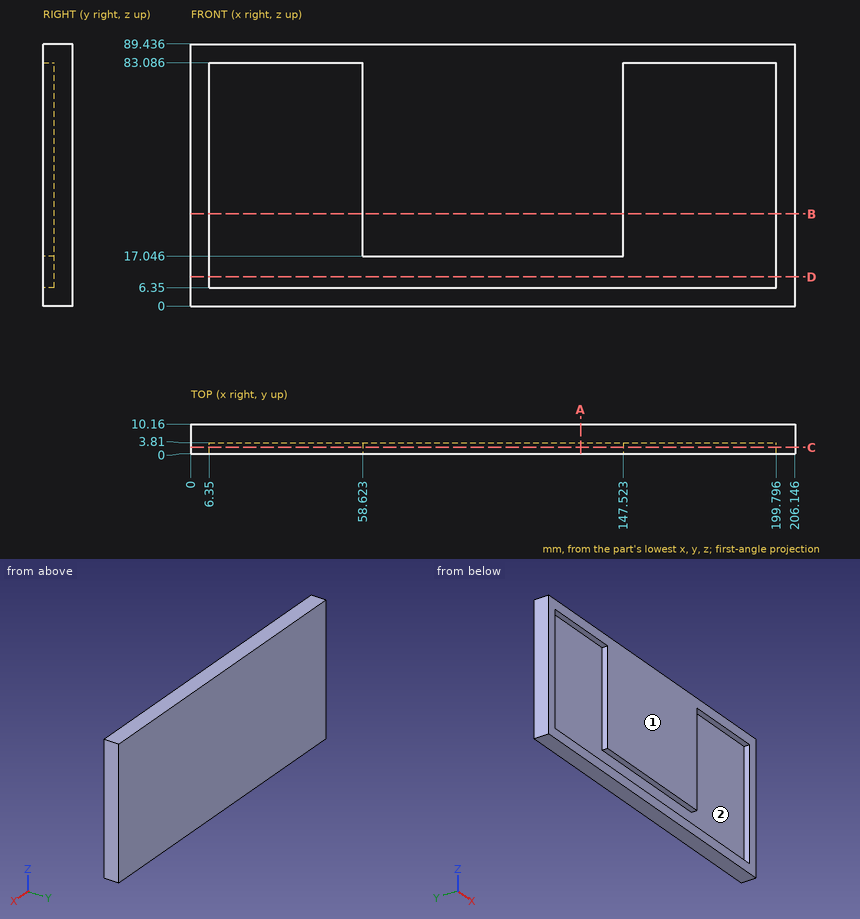
Part print with two shaded views. Sizes in mm from the minimum x, y, z corner. Give positions to 0.01 mm unless a question says otherwise; leave off trailing zeros. Order: outer loops, then holes, each group sorted by start corner. A loop starts at its lowest first (then second) coordinate and runs counter-clockwise, first axis right, second up. Notation, with made-up numbers: M 23.25,-18.5 L 69.25,-18.5 A21 cw 69.25,15.5 Z; hole C -1,6.5 d7. An arc over 180 degrees is marked long. Put each result on its own line as item: value.
Item 1: Pull direction X, two halves, no side cores. Call the marked faces 1 and 2: +X half, -X half, draft (parallel to the pull), parting line (faces both ways), or undercut.
Results are:
face 1: draft
face 2: undercut
Item 2: Drop flat-ended pins along their axis: pin 1 Ø3 at (x, y) = (104.5, 4.5) entering from -Z; pin 2 Ø3 at (x, z) = (178.5, 52) entering from -Y. Give the stop position or say it passes through.
Results are:
pin 1: z = 0
pin 2: y = 3.81
Item 3: Cut at D-D on z = 10. Write the cut outline in (x, y), then the cut area to 3 significant figures.
Results are:
outline: M 0,0 L 6.35,0 L 6.35,3.81 L 199.8,3.81 L 199.8,0 L 206.15,0 L 206.15,10.16 L 0,10.16 Z
area: 1,360 mm2
Item 4: Cut at B-B on z = 31.5. Write the cut outline in (x, y).
Results are:
outline: M 0,0 L 6.35,0 L 6.35,3.81 L 58.62,3.81 L 58.62,0 L 147.52,0 L 147.52,3.81 L 199.8,3.81 L 199.8,0 L 206.15,0 L 206.15,10.16 L 0,10.16 Z
Item 5: Cut at C-C on y = 2.25. Write the cut outline in (x, z).
Results are:
outline: M 0,0 L 206.15,0 L 206.15,89.44 L 0,89.44 Z; hole M 6.35,6.35 L 199.8,6.35 L 199.8,83.09 L 147.52,83.09 L 147.52,17.05 L 58.62,17.05 L 58.62,83.09 L 6.35,83.09 Z
Item 6: Cut at A-A on x = 133. Write the cut outline in (y, z).
Results are:
outline: M 0,0 L 10.16,0 L 10.16,89.44 L 0,89.44 L 0,17.05 L 3.81,17.05 L 3.81,6.35 L 0,6.35 Z
Item 7: Wall check: probe 1 along X at (y, z) = (1, 81); probe 2 along X at (y, z) = (3.25, 15); probe 3 along Z at (x, y) = (103.5, 3.25). Give the ranges that are in metal, low to high.
Results are:
probe 1: 0 to 6.35, 58.62 to 147.52, 199.8 to 206.15
probe 2: 0 to 6.35, 199.8 to 206.15
probe 3: 0 to 6.35, 17.05 to 89.44
